```python
from build123d import *

# Parameters (mm, degrees)
BOSS_EXTRUDE1_DEPTH = 3
SKETCH2_R           = 6.25
CUT_EXTRUDE1_DEPTH  = 6


with BuildPart() as part:
    # Sketch1 → Boss-Extrude1 (new body, symmetric)
    with BuildSketch(Plane(origin=(0, 0, 0), x_dir=(1, 0, 0), z_dir=(0, 1, 0))):
        with BuildLine():
            ThreePointArc((-96.9, 0), (-68.840352075, 70.526342596), (0, 102.5))
            ThreePointArc((0, 102.5), (70.526342596, 72.120220464), (96.9, 0))
            ThreePointArc((96.9, 0), (68.840352075, -70.526342596), (0, -102.5))
            ThreePointArc((0, -102.5), (-70.526342596, -72.120220464), (-96.9, 0))
        make_face()
    extrude(amount=BOSS_EXTRUDE1_DEPTH, both=True)

    # Sketch2 → Cut-Extrude1 (cut)
    with BuildSketch(Plane(origin=(0, 3, 0), x_dir=(1, 0, 0), z_dir=(0, 1, 0))):
        with Locations((-50, 0)):
            Circle(SKETCH2_R)
        with Locations((50, 0)):
            Circle(SKETCH2_R)
    extrude(amount=-CUT_EXTRUDE1_DEPTH, mode=Mode.SUBTRACT)


solid = part.part
```
Could you check a few things on this model? Use its own coordinates, in mm. Round coordinates to 2 decimals unless told otherwise and drop trailing zeros. Write each loop counter-clockwise with the first axis right and the second up, starting at its lowest first coordinate (ties: lowest second). Pieces come first, ordered by that corner, then holes. Notation, with made-up numbers: M 16,-5 L 75,-5 A26 cw 75,24 Z; hole C 28,-20.75 d4. An arc over 180 degrees is marked long. Answer in a Markdown table with one row per item. Add a question column.
Q1. Will this pin go through, and if not, where does the flat tip stop? pin 1 Ø3 at (y, z) = (2, -74) entering from +X.
Q2. If I drill on line 1 (X direction, y = -0.3, z = 0); line 2 (Z direction, x = 50, y = -0.55); line 3 (Z direction, x = 51, y = 0.3), over which ranges is the centre line in solid material (lowest first)? Write a range as from..to.
Q3. Imagine slicing it at C-C (z = -28.5). Please give me the cut outline in (x, y), then the cut area to 3 significant figures.
Q4. Imagine slicing it at D-D (x = -40). Please give me the cut outline in (y, z), then the cut area to 3 significant figures.
Q5. If we mould it in two halves opening along X, with no side actions, what happens to faces 1 (the cylindrical face through (69.76, 0.04, -72.92)), 2 (the flat face through (1, 3, -1)), 3 (the cylindrical face through (-44.04, 0.04, -1.88)), 4 (the cylindrical face through (55.96, 0.04, -1.88))? For each: +X half, -X half, draft (parallel to the pull), parting line (faces both ways), or undercut.
Q6. Imagine slicing it at A-A (y = 0.8). Please give me the cut outline in (x, z), then the cut area to 3 significant figures.
Q7. Imagine slicing it at B-B (x = 50). Please give me the cut outline in (y, z), then the cut area to 3 significant figures.
Values:
| question | item | result |
|---|---|---|
| 1 | pin 1 | x = 70.17 |
| 2 | line 1 | -96.9..-56.25, -43.75..43.75, 56.25..96.9 |
| 2 | line 2 | -88.63..-6.25, 6.25..86.2 |
| 2 | line 3 | -88.02..-6.17, 6.17..85.54 |
| 3 | outline | M -92.86,-3 L 94.28,-3 L 94.28,3 L -92.86,3 Z |
| 3 | area | 1,120 mm^2 |
| 4 | outline | M -3,-91.9 L 3,-91.9 L 3,93.87 L -3,93.87 Z |
| 4 | area | 1,110 mm^2 |
| 5 | face 1 | +X half |
| 5 | face 2 | draft |
| 5 | face 3 | undercut |
| 5 | face 4 | undercut |
| 6 | outline | M -96.9,0 A102.66 ccw 0,-102.5 A97.05 ccw 96.9,0 A102.66 ccw 0,102.5 A97.05 ccw Z; hole C -50,0 d12.5; hole C 50,0 d12.5 |
| 6 | area | 31,000 mm^2 |
| 7 | outline | M -3,-88.63 L 3,-88.63 L 3,-6.25 L -3,-6.25 Z; M -3,6.25 L 3,6.25 L 3,86.2 L -3,86.2 Z |
| 7 | area | 974 mm^2 |
